Check sheet for the modelled part. Datum: model origin and axes. Units: mm. A direction names the side the tool comes from. Round coordinates to 2 decimals unless told otherwise and drop trailing zeros. Write each loop counter-clockwise with the first axis right and the second up, starting at its lowest first coordinate (ties: lowest second). Pieces come first, ordered by that corner, then holes. Notation, with made-up numbers: M -13,54 L 33,54 A19 cw 33,80 Z; hole C 61,9 d6. An arc over 180 degrees is marked long. One line per item, written item: value.
from build123d import *

# Parameters (mm, degrees)
F0_R     = 16
F0_R_2   = 8.8
F1_DEPTH = 2
F2_R     = 10
F2_R_2   = 8.8
F3_DEPTH = 12
F6_DEPTH = 6.2
F9_DEPTH = 3.2
F10_SIZE = 0.6


with BuildPart() as f1:
    # F0 (on Top) → F1 (new body)
    with BuildSketch(Plane.XY):
        Circle(F0_R)
        Circle(F0_R_2, mode=Mode.SUBTRACT)
    extrude(amount=F1_DEPTH)

    # F2 (on face) → F3 (join)
    with BuildSketch(Plane.XY.offset(2)):
        Circle(F2_R)
        Circle(F2_R_2, mode=Mode.SUBTRACT)
    extrude(amount=F3_DEPTH)

    # F5 (on offset) → F6 (join, through all)
    with BuildSketch(Plane.XY.offset(7.8)):
        with BuildLine():
            Line((-2, -9.7979589711), (-2, -11.8321595662))
            ThreePointArc((-2, -11.8321595662), (0, -12), (2, -11.8321595662))
            Line((2, -11.8321595662), (2, -9.7979589711))
            ThreePointArc((2, -9.7979589711), (0, -10), (-2, -9.7979589711))
        make_face()
        with BuildLine():
            ThreePointArc((2, 11.8321595662), (0, 12), (-2, 11.8321595662))
            Line((-2, 11.8321595662), (-2, 9.7979589711))
            ThreePointArc((-2, 9.7979589711), (0, 10), (2, 9.7979589711))
            Line((2, 9.7979589711), (2, 11.8321595662))
        make_face()
    extrude(amount=F6_DEPTH)

    # F8 (on offset) → F9 (join, through all)
    with BuildSketch(Plane.XY.offset(10.8)):
        with BuildLine():
            ThreePointArc((9.1651513899, 4), (10, 0), (9.1651513899, -4))
            Line((9.1651513899, -4), (11.313708499, -4))
            ThreePointArc((11.313708499, -4), (12, 0), (11.313708499, 4))
            Line((11.313708499, 4), (9.1651513899, 4))
        make_face()
    extrude(amount=F9_DEPTH)

    # F10
    f10_edges = [f1.edges().sort_by_distance(p)[0] for p in [
        (-8.8, 0, 0),
        (-2, 10.815059, 7.8),
        (2, 10.815059, 7.8),
        (10.23943, 4, 10.8),
        (10.23943, -4, 10.8),
        (-2, -10.815059, 7.8),
        (2, -10.815059, 7.8),
    ]]
    chamfer(f10_edges, length=F10_SIZE)


solid = f1.part
Q1. Access from +Z, -Z, +X, -X, +Y, -Y to the whole of each face (thin tool, end or side, straight path). Record for faces 1 (the flat face through (2, -11, 11)), 2 (the cylindrical face through (12, 0, 12)), 3 (the flat face through (10, 4, 13)).
Completed:
face 1: +Z, +X, -Y
face 2: +Z, +X
face 3: +Z, +X, +Y
Q2. Sectioned sample at A-A on y = 0. Enter the section's corners in (x, z), and give its area (3 significant figures).
Completed:
outline: M -16,0 L -9.4,0 L -8.8,0.6 L -8.8,14 L -10,14 L -10,2 L -16,2 Z; M 8.8,0.6 L 9.4,0 L 16,0 L 16,2 L 10,2 L 10,10.8 L 12,10.8 L 12,14 L 8.8,14 Z
area: 63.6 mm^2
Q3. Sectioned sample at B-B on x = 0. Enter the section's corners in (y, z).
Completed:
outline: M -16,0 L -9.4,0 L -8.8,0.6 L -8.8,14 L -12,14 L -12,7.8 L -10,7.8 L -10,2 L -16,2 Z; M 8.8,0.6 L 9.4,0 L 16,0 L 16,2 L 10,2 L 10,7.8 L 12,7.8 L 12,14 L 8.8,14 Z
Q4. Scan lines: line 1 (Y direction, x = 0, z = 4); line 2 (Z direction, x = 11, y = 0.5); line 3 (Z direction, x = 9.5, y = -4.5). Record each from-to range of solid material in increasing order. Write a range as [from, to].
Completed:
line 1: [-10, -8.8], [8.8, 10]
line 2: [0, 2], [10.8, 14]
line 3: [0, 2]
Q5. Depth check by flat-ended pin: P1, Ø1, axis at y = -10.5, z = 12, coming from the -X side; P2, Ø9.5, axis at x = -0.5, y = 2, coming from the +Z side; P3, Ø6, axis at x = 7, z = 12.5, coming from the -Y side; P4, Ø2, axis at y = 11, z = 11.5, coming from the +X side. Enter the tip coordinate at first touch or a pass-through.
Completed:
P1: x = -2
P2: through
P3: y = -9.17
P4: x = 2
Q6. Sectioned sample at C-C on z = 10.25. Enter the section's corners in (x, y).
Completed:
outline: M -2,-11.83 A12 ccw 2,-11.83 L 2,-9.8 A10 ccw 2,9.8 L 2,11.83 A12 ccw -2,11.83 L -2,9.8 A10 ccw -2,-9.8 Z; hole C 0,0 d17.6
Q7. Sectioned sample at D-D on x = 10.5. Enter the section's corners in (y, z).
Completed:
outline: M -12.07,0 L 12.07,0 L 12.07,2 L -12.07,2 Z; M -4,11.4 L -3.4,10.8 L 3.4,10.8 L 4,11.4 L 4,14 L -4,14 Z
